The model under review builds one solid part; all positions refer to its coordinate system, in mm. A direction names the side the tool comes from. Give positions to 0.01 mm unless a question says otherwise; leave off trailing zeros. Loops run counter-clockwise (first coordinate to the right, second up) from the corner with the lowest first, then second, coordinate; pieces in that order, holes last. Notation, with made-up numbers: (83, 51) - (89, 51) arc R32 ccw to (89, 88) - close; hole circle Ø11 at (89, 56.5). An arc over 180 degrees is marked (long way). Answer as a JSON object with one key per item and string values.
from build123d import *

# Parameters (mm, degrees)
F0_R     = 14
F1_DEPTH = 20
F2_R     = 5.8
F3_DEPTH = 20.001
F5_DEPTH = 5
F6_DEPTH = 5
F7_DEPTH = 5
F9_DEPTH = 4


with BuildPart() as f1:
    # F0 (on Top) → F1 (new body)
    with BuildSketch(Plane.XY):
        Circle(F0_R)
    extrude(amount=F1_DEPTH)

    # F2 (on face) → F3 (cut, through all)
    with BuildSketch(Plane(origin=(0, 0, 0), x_dir=(1, 0, 0), z_dir=(0, 0, -1))):
        Circle(F2_R)
    extrude(amount=-F3_DEPTH, mode=Mode.SUBTRACT)

    # F4 (on face) → F5 (cut)
    with BuildSketch(Plane.XY.offset(20)):
        with BuildLine():
            Line((-2.5, 5.2335456433), (-2.5, 13.774977314))
            ThreePointArc((-2.5, 13.774977314), (-14, 0), (-2.5, -13.774977314))
            Line((-2.5, -13.774977314), (-2.5, -5.2335456433))
            ThreePointArc((-2.5, -5.2335456433), (-5.8, 0), (-2.5, 5.2335456433))
        make_face()
    extrude(amount=-F5_DEPTH, mode=Mode.SUBTRACT)

    # F4 (on face) → F6 (cut)
    with BuildSketch(Plane.XY.offset(20)):
        with BuildLine():
            ThreePointArc((14, 0), (10.7470926301, 8.9721792225), (2.5, 13.774977314))
            Line((2.5, 13.774977314), (2.5, 5.2335456433))
            ThreePointArc((2.5, 5.2335456433), (4.9061186288, 3.0935416597), (5.8, 0))
            ThreePointArc((5.8, 0), (4.9061186288, -3.0935416597), (2.5, -5.2335456433))
            Line((2.5, -5.2335456433), (2.5, -13.774977314))
            ThreePointArc((2.5, -13.774977314), (10.7470926301, -8.9721792225), (14, 0))
        make_face()
    extrude(amount=-F6_DEPTH, mode=Mode.SUBTRACT)

    # F4 (on face) → F7 (join)
    with BuildSketch(Plane.XY.offset(20)):
        with BuildLine():
            Line((2.5, -13.774977314), (2.5, -5.2335456433))
            ThreePointArc((2.5, -5.2335456433), (0, -5.8), (-2.5, -5.2335456433))
            Line((-2.5, -5.2335456433), (-2.5, -13.774977314))
            ThreePointArc((-2.5, -13.774977314), (0, -14), (2.5, -13.774977314))
        make_face()
    extrude(amount=F7_DEPTH)

    # F8 (on face) → F9 (cut)
    with BuildSketch(Plane.XY.offset(25)):
        with BuildLine():
            Line((-2.5, -5.2335456433), (-2.5, -10))
            Line((-2.5, -10), (2.5, -10))
            Line((2.5, -10), (2.5, -5.2335456433))
            ThreePointArc((2.5, -5.2335456433), (0, -5.8), (-2.5, -5.2335456433))
        make_face()
    extrude(amount=-F9_DEPTH, mode=Mode.SUBTRACT)


solid = f1.part
Q1. Consider section B-B, the plane z = 16.5. State the section outline as (x, y) points, plus the area to 3 significant figures.
Results:
{"outline": "(-2.5, -13.77) arc R14 ccw to (2.5, -13.77) - (2.5, -5.23) arc R5.8 cw to (-2.5, -5.23) - close; (-2.5, 5.23) arc R5.8 cw to (2.5, 5.23) - (2.5, 13.77) arc R14 ccw to (-2.5, 13.77) - close", "area": "83.1 mm^2"}
Q2. Clearance check with flat-ended pins moving along their axes: pin 1 Ø5 at (x, z) = (8, 19.5) entering from -Y; pin 2 Ø1.4 at (x, y) = (1, -7.5) entering from +Z; pin 3 Ø4.5 at (y, z) = (-11.5, 18) entering from -X; pin 4 Ø2 at (y, z) = (-5, 21.5) entering from +X. State where each tip first meets the part, or that it passes through.
Results:
{"pin 1": "passes through", "pin 2": "stops at z = 21", "pin 3": "stops at x = -2.5", "pin 4": "stops at x = 2.5"}
Q3. For faces 1 (the face through (0, -6, 0)), 2 (the face through (-2.5, 9, 18)), 3 (the face through (8, 0, 15)), 4 (the face through (0, 10, 20)), 5 (the face through (0, -12, 25)), list the 3-axis set-ups (+Z, -Z, +X, -X, +Y, -Y) from which the entire face can be reached by the end or side of a thin tool; tool diameter is ignored.
Results:
{"face 1": "-Z, +X, -X, +Y, -Y", "face 2": "+Z, -X, +Y, -Y", "face 3": "+Z, +X, +Y, -Y", "face 4": "+Z, +X, -X, +Y", "face 5": "+Z, +X, -X, +Y, -Y"}
Q4. Consider section D-D, the plane z = 9.75. State the section outline as (x, y) points.
Results:
{"outline": "circle Ø28 at (0, 0); hole circle Ø11.6 at (0, 0)"}
Q5. To check wall thickness, follow probe 1 along Y at (x, z) = (0, 5); probe 2 along Z at (x, y) = (-12, 4.25). State the ranges of each line that lie inside material, in increasing order. Write a range as [from, to].
Results:
{"probe 1": "y = [-14, -5.8], [5.8, 14]", "probe 2": "z = [0, 15]"}
Q6. Consider section C-C, the plane x = 0. State the section outline as (y, z) points, plus the area to 3 significant figures.
Results:
{"outline": "(-14, 0) - (-5.8, 0) - (-5.8, 21) - (-10, 21) - (-10, 25) - (-14, 25) - close; (5.8, 0) - (14, 0) - (14, 20) - (5.8, 20) - close", "area": "352 mm^2"}
Q7. Consider section A-A, the plane y = 0. State the section outline as (x, z) points, plus the area to 3 significant figures.
Results:
{"outline": "(-14, 0) - (-5.8, 0) - (-5.8, 15) - (-14, 15) - close; (5.8, 0) - (14, 0) - (14, 15) - (5.8, 15) - close", "area": "246 mm^2"}
